Autodesk Inventor part; units mm, degrees
ref_plane "YZ Plane" through (0, 0, 0) normal (1, 0, 0) x (0, 1, 0)
ref_plane "XZ Plane" through (0, 0, 0) normal (0, 1, 0) x (-1, 0, 0)
ref_plane "XY Plane" through (0, 0, 0) normal (0, 0, 1) x (1, 0, 0)
sketch "Sketch1" plane through (0, 0, 0) normal (0, 0, 1) x (1, 0, 0)
  circle A0 centre (0, 0) radius 17.4625
  dimension "d0" = 34.925
extrude "Extrusion1" add sketch "Sketch1" along normal mid plane 99.06
sketch "Sketch2" plane through (0, 0, 49.53) normal (0, 0, 1) x (1, 0, 0)
  circle A0 centre (0, 0) radius 15.9385
  circle A1 centre (0, 0) radius 17.4625
  dimension "d16" = 1.524
extrude "Extrusion2" cut sketch "Sketch2" against normal blind 99.06 contours A0
sketch "Sketch3" plane through (0, 0, 0) normal (0, 0, 1) x (1, 0, 0)
  circle A0 centre (0, 0) radius 17.3355
  circle A1 centre (0, 0) radius 17.4625
  dimension "d6" = 34.671
extrude "Extrusion3" cut sketch "Sketch3" along normal mid plane 3.9688
pattern_linear "Rectangular Pattern1" count 3 spacing 16.129 along (0, 0, 1) count 3 spacing 16.129 along (0, 0, -1) of "Extrusion3"
properties part number "MIddle Rod Cover" material "Stainless Steel"
CAD build for the part. Positions are in the model's coordinates, mm. A direction names the side the tool comes from. Give positions to 0.01 mm unless a question says otherwise; leave off trailing zeros. Write each loop counter-clockwise with the first axis right and the second up, starting at its lowest first coordinate (ties: lowest second). Pieces come first, ordered by that corner, then holes. Notation, with made-up numbers: (12, 53.25) -> (47, 53.25) arc R22 ccw to (47, 63.25) -> close; hole circle Ø11 at (40.5, 38.5). An arc over 180 degrees is marked (long way). Return JSON: item names as keys, results as strings.
Item 1: Drop flat-ended pins along their axis: pin 1 (2 mm diameter, centred on x = 10.5, z = -36.5, fed in from +Y); pin 2 (1 mm diameter, centred on x = -8, z = -5.5, fed in from +Y); pin 3 (10 mm diameter, centred on y = 10.5, z = -38.5, fed in from +X). Give the stop position or say it passes through.
Answer below:
{"pin 1": "stops at y = 14.65", "pin 2": "stops at y = 15.77", "pin 3": "stops at x = 16.57"}
Item 2: Tool access for faces 1 (the cylindrical face through (-13.858, 10.626, 41.779)), 2 (the cylindrical face through (-17.32, 0.76, 32.29)): list every direction of +Z, -Z, +X, -X, +Y, -Y with a clear straight run to the whole face (end or side of a thin tool).
Answer below:
{"face 1": "+Z, -Z", "face 2": "none"}
Item 3: Band-saw the part on A-A (z = 5.5). List the corners of the cut face in (x, y) (1 decimal).
Answer below:
{"outline": "circle Ø34.9 at (0, 0); hole circle Ø31.9 at (0, 0)"}
Item 4: Two-plate mould, pull along Z, no slides. Class faces 3 (the cylindrical face through (-13.858, -10.626, -24.108)), 4 (the cylindrical face through (-17.32, 0.76, 0.03)), 5 (the flat face through (8, -14, -49.53)): +Z half, -Z half, draft (parallel to the pull), parting line (faces both ways), or undercut.
Answer below:
{"face 3": "draft", "face 4": "undercut", "face 5": "-Z half"}
Item 5: Drill centre lines: probe 1 along Y at (x, z) = (0, 23.5); probe 2 along Y at (x, z) = (8, 5.5); probe 3 along X at (y, z) = (-9, 15). Where is each one in solid material? Low to high.
Answer below:
{"probe 1": "y = -17.46 to -15.94, 15.94 to 17.46", "probe 2": "y = -15.52 to -13.79, 13.79 to 15.52", "probe 3": "x = -14.82 to -13.15, 13.15 to 14.82"}
